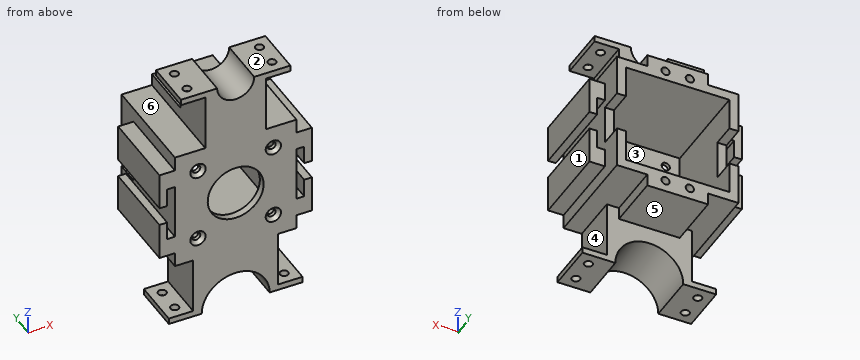
from build123d import *

# Parameters (mm, degrees)
SKETCH1_W                                    = 50
SKETCH1_H                                    = 50
BOSS_EXTRUDE1_DEPTH                          = 3
SKETCH3_W                                    = 50
SKETCH3_H                                    = 50
SKETCH3_W_2                                  = 42.5
SKETCH3_H_2                                  = 42.5
BOSS_EXTRUDE2_DEPTH                          = 39.7
SKETCH9_W                                    = 25
SKETCH9_H                                    = 20
BOSS_EXTRUDE4_DEPTH                          = 25.8
CUT_EXTRUDE1_REACH                           = 62.999
SKETCH11_R                                   = 7.62
SKETCH12_W                                   = 2.5
SKETCH12_H                                   = 20
BOSS_EXTRUDE5_DEPTH                          = 10
CUT_EXTRUDE2_REACH                           = 92.52
SKETCH13_R                                   = 1.7
SKETCH15_W                                   = 35
SKETCH15_H                                   = 20
BOSS_EXTRUDE6_DEPTH                          = 25.8
CUT_EXTRUDE3_REACH                           = 62.999
SKETCH16_R                                   = 13.97
SKETCH17_W                                   = 2.5
SKETCH17_H                                   = 20
BOSS_EXTRUDE7_DEPTH                          = 10
CUT_EXTRUDE4_REACH                           = 115.587
SKETCH18_R                                   = 1.7
CUT_EXTRUDE5_START                           = -5
SKETCH19_W                                   = 16.15
SKETCH19_H                                   = 9.6
CUT_EXTRUDE5_DEPTH                           = 90.617846817
SKETCH20_W                                   = 25
SKETCH20_H                                   = 5
BOSS_EXTRUDE8_DEPTH                          = 22.7
SKETCH21_R                                   = 1.7
CUT_EXTRUDE6_DEPTH                           = 10
SKETCH23_W                                   = 7.62
SKETCH23_H                                   = 33.09
BOSS_EXTRUDE9_DEPTH                          = 6.35
SKETCH24_W                                   = 3.175
SKETCH24_H                                   = 33.09
BOSS_EXTRUDE10_DEPTH                         = 7.62
SKETCH25_W                                   = 3.175
SKETCH25_H                                   = 33.09
BOSS_EXTRUDE11_DEPTH                         = 7.62
CUT_EXTRUDE8_REACH                           = 75.394
SKETCH27_R                                   = 11.5
CSK_FOR_M3_COUNTERSUNK_FLAT_HEAD_SCR_2_COUNT = 2
CSK_FOR_M3_COUNTERSUNK_FLAT_HEAD_SCR_2_PITCH = 31
CSK_FOR_M3_COUNTERSUNK_FLAT_HEAD_SCR_3_COUNT = 2
CSK_FOR_M3_COUNTERSUNK_FLAT_HEAD_SCR_3_PITCH = 43.840620434
CSK_FOR_M3_COUNTERSUNK_FLAT_HEAD_SCR_4_COUNT = 2
CSK_FOR_M3_COUNTERSUNK_FLAT_HEAD_SCR_4_PITCH = 31


with BuildPart() as part:
    # Sketch1 → Boss-Extrude1 (new body)
    with BuildSketch(Plane(origin=(0, 0, 0), x_dir=(1, 0, 0), z_dir=(0, 1, 0))):
        Rectangle(SKETCH1_W, SKETCH1_H)
    extrude(amount=BOSS_EXTRUDE1_DEPTH)

    # Sketch3 → Boss-Extrude2 (add)
    with BuildSketch(Plane(origin=(0, 3, 0), x_dir=(1, 0, 0), z_dir=(0, 1, 0))):
        Rectangle(SKETCH3_W, SKETCH3_H)
        Rectangle(SKETCH3_W_2, SKETCH3_H_2, mode=Mode.SUBTRACT)
    extrude(amount=BOSS_EXTRUDE2_DEPTH)

    # Sketch9 → Boss-Extrude4 (add)
    with BuildSketch(Plane.XY.offset(25)):
        with Locations((0, 10)):
            Rectangle(SKETCH9_W, SKETCH9_H)
    extrude(amount=BOSS_EXTRUDE4_DEPTH)

    # Sketch11 → Cut-Extrude1 (cut, up to next)
    with BuildSketch(Plane(origin=(0, 20, 0), x_dir=(1, 0, 0), z_dir=(0, 1, 0)), mode=Mode.PRIVATE) as cut_extrude1_sk1:
        with Locations((0, -50.8)):
            Circle(SKETCH11_R)
    cut_extrude1_tool1 = extrude(cut_extrude1_sk1.sketch, amount=-CUT_EXTRUDE1_REACH, mode=Mode.PRIVATE) & part.part
    add(cut_extrude1_tool1.solids().sort_by_distance((0, 20, 50.8))[0], mode=Mode.SUBTRACT)

    # Sketch12 → Boss-Extrude5 (add)
    with BuildSketch(Plane.ZY.offset(12.5)):
        with Locations((49.55, 10)):
            Rectangle(SKETCH12_W, SKETCH12_H)
    boss_extrude5 = extrude(amount=BOSS_EXTRUDE5_DEPTH)

    # Mirror2: Boss-Extrude5 across plane
    add(boss_extrude5.mirror(Plane(origin=(0, 0, 0), x_dir=(0, 0, 1), z_dir=(1, 0, 0))))

    # Sketch13 → Cut-Extrude2 (cut, up to next)
    with BuildSketch(Plane.XY.offset(50.8), mode=Mode.PRIVATE) as cut_extrude2_sk1:
        with Locations((-17.5, 5)):
            Circle(SKETCH13_R)
    cut_extrude2_tool1 = extrude(cut_extrude2_sk1.sketch, amount=-CUT_EXTRUDE2_REACH, mode=Mode.PRIVATE) & part.part
    # Sketch13 → Cut-Extrude2 (cut, up to next)
    with BuildSketch(Plane.XY.offset(50.8), mode=Mode.PRIVATE) as cut_extrude2_sk2:
        with Locations((17.5, 5)):
            Circle(SKETCH13_R)
    cut_extrude2_tool2 = extrude(cut_extrude2_sk2.sketch, amount=-CUT_EXTRUDE2_REACH, mode=Mode.PRIVATE) & part.part
    # Sketch13 → Cut-Extrude2 (cut, up to next)
    with BuildSketch(Plane.XY.offset(50.8), mode=Mode.PRIVATE) as cut_extrude2_sk3:
        with Locations((-17.5, 15)):
            Circle(SKETCH13_R)
    cut_extrude2_tool3 = extrude(cut_extrude2_sk3.sketch, amount=-CUT_EXTRUDE2_REACH, mode=Mode.PRIVATE) & part.part
    # Sketch13 → Cut-Extrude2 (cut, up to next)
    with BuildSketch(Plane.XY.offset(50.8), mode=Mode.PRIVATE) as cut_extrude2_sk4:
        with Locations((17.5, 15)):
            Circle(SKETCH13_R)
    cut_extrude2_tool4 = extrude(cut_extrude2_sk4.sketch, amount=-CUT_EXTRUDE2_REACH, mode=Mode.PRIVATE) & part.part
    add(cut_extrude2_tool1.solids().sort_by_distance((-17.5, 5, 50.8))[0], mode=Mode.SUBTRACT)
    add(cut_extrude2_tool2.solids().sort_by_distance((17.5, 5, 50.8))[0], mode=Mode.SUBTRACT)
    add(cut_extrude2_tool3.solids().sort_by_distance((-17.5, 15, 50.8))[0], mode=Mode.SUBTRACT)
    add(cut_extrude2_tool4.solids().sort_by_distance((17.5, 15, 50.8))[0], mode=Mode.SUBTRACT)

    # Sketch15 → Boss-Extrude6 (add)
    with BuildSketch(Plane(origin=(0, 0, -25), x_dir=(-1, 0, 0), z_dir=(0, 0, -1))):
        with Locations((0, 10)):
            Rectangle(SKETCH15_W, SKETCH15_H)
    extrude(amount=BOSS_EXTRUDE6_DEPTH)

    # Sketch16 → Cut-Extrude3 (cut, up to next)
    with BuildSketch(Plane(origin=(0, 20, 0), x_dir=(1, 0, 0), z_dir=(0, 1, 0)), mode=Mode.PRIVATE) as cut_extrude3_sk1:
        with Locations((0, 50.8)):
            Circle(SKETCH16_R)
    cut_extrude3_tool1 = extrude(cut_extrude3_sk1.sketch, amount=-CUT_EXTRUDE3_REACH, mode=Mode.PRIVATE) & part.part
    add(cut_extrude3_tool1.solids().sort_by_distance((0, 20, -50.8))[0], mode=Mode.SUBTRACT)

    # Sketch17 → Boss-Extrude7 (add)
    with BuildSketch(Plane.ZY.offset(17.5)):
        with Locations((-49.55, 10)):
            Rectangle(SKETCH17_W, SKETCH17_H)
    boss_extrude7 = extrude(amount=BOSS_EXTRUDE7_DEPTH)

    # Mirror3: Boss-Extrude7 across plane
    add(boss_extrude7.mirror(Plane(origin=(0, 0, 0), x_dir=(0, 0, 1), z_dir=(1, 0, 0))))

    # Sketch18 → Cut-Extrude4 (cut, up to next)
    with BuildSketch(Plane(origin=(0, 0, -50.8), x_dir=(-1, 0, 0), z_dir=(0, 0, -1)), mode=Mode.PRIVATE) as cut_extrude4_sk1:
        with Locations((-22.5, 15)):
            Circle(SKETCH18_R)
    cut_extrude4_tool1 = extrude(cut_extrude4_sk1.sketch, amount=-CUT_EXTRUDE4_REACH, mode=Mode.PRIVATE) & part.part
    # Sketch18 → Cut-Extrude4 (cut, up to next)
    with BuildSketch(Plane(origin=(0, 0, -50.8), x_dir=(-1, 0, 0), z_dir=(0, 0, -1)), mode=Mode.PRIVATE) as cut_extrude4_sk2:
        with Locations((-22.5, 5)):
            Circle(SKETCH18_R)
    cut_extrude4_tool2 = extrude(cut_extrude4_sk2.sketch, amount=-CUT_EXTRUDE4_REACH, mode=Mode.PRIVATE) & part.part
    # Sketch18 → Cut-Extrude4 (cut, up to next)
    with BuildSketch(Plane(origin=(0, 0, -50.8), x_dir=(-1, 0, 0), z_dir=(0, 0, -1)), mode=Mode.PRIVATE) as cut_extrude4_sk3:
        with Locations((22.5, 15)):
            Circle(SKETCH18_R)
    cut_extrude4_tool3 = extrude(cut_extrude4_sk3.sketch, amount=-CUT_EXTRUDE4_REACH, mode=Mode.PRIVATE) & part.part
    # Sketch18 → Cut-Extrude4 (cut, up to next)
    with BuildSketch(Plane(origin=(0, 0, -50.8), x_dir=(-1, 0, 0), z_dir=(0, 0, -1)), mode=Mode.PRIVATE) as cut_extrude4_sk4:
        with Locations((22.5, 5)):
            Circle(SKETCH18_R)
    cut_extrude4_tool4 = extrude(cut_extrude4_sk4.sketch, amount=-CUT_EXTRUDE4_REACH, mode=Mode.PRIVATE) & part.part
    add(cut_extrude4_tool1.solids().sort_by_distance((22.5, 15, -50.8))[0], mode=Mode.SUBTRACT)
    add(cut_extrude4_tool2.solids().sort_by_distance((22.5, 5, -50.8))[0], mode=Mode.SUBTRACT)
    add(cut_extrude4_tool3.solids().sort_by_distance((-22.5, 15, -50.8))[0], mode=Mode.SUBTRACT)
    add(cut_extrude4_tool4.solids().sort_by_distance((-22.5, 5, -50.8))[0], mode=Mode.SUBTRACT)

    # Sketch19 → Cut-Extrude5 (cut)
    with BuildSketch(Plane(origin=(25, 0, 0), x_dir=(0, 0, -1), z_dir=(1, 0, 0)).offset(CUT_EXTRUDE5_START)):
        with Locations((0, 37.9)):
            Rectangle(SKETCH19_W, SKETCH19_H)
    cut_extrude5 = extrude(amount=CUT_EXTRUDE5_DEPTH, mode=Mode.SUBTRACT)

    # Sketch20 → Boss-Extrude8 (add)
    with BuildSketch(Plane(origin=(0, 20, 0), x_dir=(1, 0, 0), z_dir=(0, 1, 0))):
        with Locations((0, -27.5)):
            Rectangle(SKETCH20_W, SKETCH20_H)
        with Locations((0, 27.5)):
            Rectangle(SKETCH20_W, SKETCH20_H)
    extrude(amount=BOSS_EXTRUDE8_DEPTH)

    # Sketch21 → Cut-Extrude6 (cut)
    with BuildSketch(Plane(origin=(0, 42.7, 0), x_dir=(1, 0, 0), z_dir=(0, 1, 0))):
        with Locations(Location((5, -25.25, 0), (0, 0, 270))):
            Circle(SKETCH21_R)
        with Locations(Location((-5, 25.25, 0), (0, 0, 270))):
            Circle(SKETCH21_R)
        with Locations(Location((5, 25.25, 0), (0, 0, 270))):
            Circle(SKETCH21_R)
        with Locations(Location((-5, -25.25, 0), (0, 0, 270))):
            Circle(SKETCH21_R)
    extrude(amount=-CUT_EXTRUDE6_DEPTH, mode=Mode.SUBTRACT)

    # Sketch23 → Boss-Extrude9 (add)
    with BuildSketch(Plane.ZY.offset(25)):
        with Locations((-15.24, 16.545)):
            Rectangle(SKETCH23_W, SKETCH23_H)
        with Locations((15.24, 16.545)):
            Rectangle(SKETCH23_W, SKETCH23_H)
    boss_extrude9 = extrude(amount=BOSS_EXTRUDE9_DEPTH)

    # Sketch24 → Boss-Extrude10 (add)
    with BuildSketch(Plane.XY.offset(-11.43)):
        with Locations((-29.7625, 16.545)):
            Rectangle(SKETCH24_W, SKETCH24_H)
    boss_extrude10 = extrude(amount=BOSS_EXTRUDE10_DEPTH)

    # Sketch25 → Boss-Extrude11 (add)
    with BuildSketch(Plane(origin=(0, 0, 11.43), x_dir=(-1, 0, 0), z_dir=(0, 0, -1))):
        with Locations((29.7625, 16.545)):
            Rectangle(SKETCH25_W, SKETCH25_H)
    boss_extrude11 = extrude(amount=BOSS_EXTRUDE11_DEPTH)

    # Sketch27 → Cut-Extrude8 (cut, up to next)
    with BuildSketch(Plane.XZ, mode=Mode.PRIVATE) as cut_extrude8_sk1:
        with Locations(Location((0, 0, 0), (0, 0, 270))):
            Circle(SKETCH27_R)
    cut_extrude8_tool1 = extrude(cut_extrude8_sk1.sketch, amount=-CUT_EXTRUDE8_REACH, mode=Mode.PRIVATE) & part.part
    add(cut_extrude8_tool1.solids().sort_by_distance((0, 0, 0))[0], mode=Mode.SUBTRACT)

    # Sketch30 → CSK for M3 Countersunk Flat Head Screw1 (revolve, cut)
    with BuildSketch(Plane(origin=(-15.5, 0, 15.5), x_dir=(0, 0, -1), z_dir=(1, 0, 0))):
        Polygon((0, 0), (0, 3), (1.7, 3), (1.7, 1.45), (3.15, 0), align=None)
    csk_for_m3_countersunk_flat_head_screw1 = revolve(axis=Axis((-15.5, -6.35, 15.5), (0, 1, 0)), mode=Mode.SUBTRACT)

    # CSK for M3 Countersunk Flat Head Scr 2: CSK for M3 Countersunk Flat Head Screw1 ×2
    with Locations(*[(i * CSK_FOR_M3_COUNTERSUNK_FLAT_HEAD_SCR_2_PITCH, 0, 0) for i in range(1, CSK_FOR_M3_COUNTERSUNK_FLAT_HEAD_SCR_2_COUNT)]):
        add(csk_for_m3_countersunk_flat_head_screw1, mode=Mode.SUBTRACT)

    # CSK for M3 Countersunk Flat Head Scr 3: CSK for M3 Countersunk Flat Head Screw1 ×2
    with Locations(*[Vector(0.7071067811865475, 0, -0.7071067811865476) * (i * CSK_FOR_M3_COUNTERSUNK_FLAT_HEAD_SCR_3_PITCH) for i in range(1, CSK_FOR_M3_COUNTERSUNK_FLAT_HEAD_SCR_3_COUNT)]):
        add(csk_for_m3_countersunk_flat_head_screw1, mode=Mode.SUBTRACT)

    # CSK for M3 Countersunk Flat Head Scr 4: CSK for M3 Countersunk Flat Head Screw1 ×2
    with Locations(*[(0, 0, -i * CSK_FOR_M3_COUNTERSUNK_FLAT_HEAD_SCR_4_PITCH) for i in range(1, CSK_FOR_M3_COUNTERSUNK_FLAT_HEAD_SCR_4_COUNT)]):
        add(csk_for_m3_countersunk_flat_head_screw1, mode=Mode.SUBTRACT)

    # Mirror4: Cut-Extrude5, Boss-Extrude9, Boss-Extrude10, Boss-Extrude11 across plane
    add(cut_extrude5.mirror(Plane(origin=(0, 0, 0), x_dir=(0, 0, 1), z_dir=(1, 0, 0))), mode=Mode.SUBTRACT)
    add(boss_extrude9.mirror(Plane(origin=(0, 0, 0), x_dir=(0, 0, 1), z_dir=(1, 0, 0))))
    add(boss_extrude10.mirror(Plane(origin=(0, 0, 0), x_dir=(0, 0, 1), z_dir=(1, 0, 0))))
    add(boss_extrude11.mirror(Plane(origin=(0, 0, 0), x_dir=(0, 0, 1), z_dir=(1, 0, 0))))


solid = part.part
Build history of the part. All positions in model axes, mm. Face numbers are marked on the shaded views. A direction names the side the tool comes from. Round coordinates to 2 decimals unless told otherwise and drop trailing zeros. Write each loop counter-clockwise with the first axis right and the second up, starting at its lowest first coordinate (ties: lowest second). Pieces come first, ordered by that corner, then holes. Notation, with made-up numbers: M 19,72.25 L 24,72.25 A15 ccw 24,99.25 Z; hole C -22,89.5 d7. An arc over 180 degrees is marked long. Use CSV: the item, a comma, the result in double quotes.
1. Wall check: probe 1 along X at (y, z) = (38, -25.25); probe 2 along Z at (x, y) = (-15.5, 1.95); probe 3 along Y at (x, z) = (22.5, -49.5). Give the ranges that are in metal, low to high. Write a range as from..to.
Reply:
probe 1,"x = -12.5..-6.7, -3.3..3.3, 6.7..12.5"
probe 2,"z = -50.8..-17.2, -13.8..13.8, 17.2..25, 48.3..50.8"
probe 3,"y = 0..3.3, 6.7..13.3, 16.7..20"
2. Saw through at B-B (z = -15.5). Give the cut face in (x, y).
Reply:
outline,"M -31.35,0 L -18.65,0 L -17.2,1.45 L -17.2,3 L -21.25,3 L -21.25,42.7 L -25,42.7 L -25,33.09 L -31.35,33.09 Z; M -13.8,1.45 L -12.35,0 L 12.35,0 L 13.8,1.45 L 13.8,3 L -13.8,3 Z; M 17.2,1.45 L 18.65,0 L 31.35,0 L 31.35,33.09 L 25,33.09 L 25,42.7 L 21.25,42.7 L 21.25,3 L 17.2,3 Z"
3. Two-plate mould, pull along Z, no slides. Class the marked faces 1, 2 and 3: +Z half, -Z half, draft (parallel to the pull), parting line (faces both ways), or undercut.
Reply:
face 1,"draft"
face 2,"+Z half"
face 3,"undercut"
4. Flat gauge pins, fed straight in: pin 1 (3 mm diameter, centred on x = 29.5, y = 16, fed in from +Z); pin 2 (1.5 mm diameter, centred on x = 16, y = 38.5, fed in from +Z); pin 3 (7 mm diameter, centred on x = -28, y = 24.5, fed in from -Z). Where does each tip first touch, or does it go through?
Reply:
pin 1,"stops at z = 19.05"
pin 2,"stops at z = 25"
pin 3,"stops at z = -25"
5. Saw through at C-C (y = 15). State how many separate pieces and enclosed holes the cut face has, plus the area to 3 significant figures.
Reply:
separate pieces,"5"
enclosed holes,"1"
area,"2,200 mm²"
6. Tool access for the marked faces 4, 5 and 6: list every direction of +Z, -Z, +X, -X, +Y, -Y with a clear straight run to the whole face (end or side of a thin tool).
Reply:
face 4,"+X, +Y, -Y"
face 5,"-Z, +X, -X, +Y"
face 6,"-X, +Y, -Y"
7. Saw through at D-D (z = -5). Give the cut face in (x, y) (3 decimals).
Reply:
outline,"M -31.35,0 L -28.175,0 L -28.175,33.09 L -31.35,33.09 Z; M -25,0 L -10.356,0 L -10.356,3 L -21.25,3 L -21.25,33.1 L -25,33.1 Z; M 10.356,0 L 25,0 L 25,33.1 L 21.25,33.1 L 21.25,3 L 10.356,3 Z; M 28.175,0 L 31.35,0 L 31.35,33.09 L 28.175,33.09 Z"
8. Saw through at A-A (x = 0). Give the cut face in (y, z).
Reply:
outline,"M 0,-36.83 L 20,-36.83 L 20,-30 L 42.7,-30 L 42.7,-21.25 L 3,-21.25 L 3,-11.5 L 0,-11.5 Z; M 0,11.5 L 3,11.5 L 3,21.25 L 42.7,21.25 L 42.7,30 L 20,30 L 20,43.18 L 0,43.18 Z"
